The model under review builds one solid part; all positions refer to its coordinate system, in mm. Face numbers are marked on the shaded views. A direction names the side the tool comes from. Give positions to 0.01 mm unless a question says otherwise; leave off trailing zeros. Loops run counter-clockwise (first coordinate to the right, second up) from the corner with the lowest first, then second, coordinate; pieces in that order, holes last. Notation, with made-up numbers: M 10.5,-2 L 33.5,-2 A17 ccw 33.5,22 Z; hole C 46,64 d6. An arc over 180 degrees is marked long. Return JSON: item names as keys, results as strings. Group by question number.
```python
from build123d import *

# Parameters (mm, degrees)
F0_W     = 127
F0_H     = 127
F1_DEPTH = 6.35
F4_DEPTH = 762


with BuildPart() as f1:
    # F0 (on Front) → F1 (new body)
    with BuildSketch(Plane.XZ):
        with Locations((5.181599, -1.836989)):
            Rectangle(F0_W, F0_H)
    extrude(amount=F1_DEPTH)

    # F3 (on face) → F4 (join)
    with BuildSketch(Plane(origin=(0, 0, 0), x_dir=(-1, 0, 0), z_dir=(0, 1, 0))):
        Polygon((-11.394211, -37.070461), (1.031012, -37.070461), (12.706903, -32.820784), (22.225176, -24.834005), (28.437787, -14.073446), (30.595405, -1.836989), (28.437787, 10.399467), (22.225176, 21.160026), (12.706903, 29.146805), (1.031012, 33.396482), (-11.394211, 33.396482), (-23.070102, 29.146805), (-32.588375, 21.160026), (-38.800986, 10.399467), (-40.958604, -1.836989), (-38.800986, -14.073446), (-32.588375, -24.834005), (-23.070102, -32.820784), align=None)
    extrude(amount=F4_DEPTH)


solid = f1.part
```
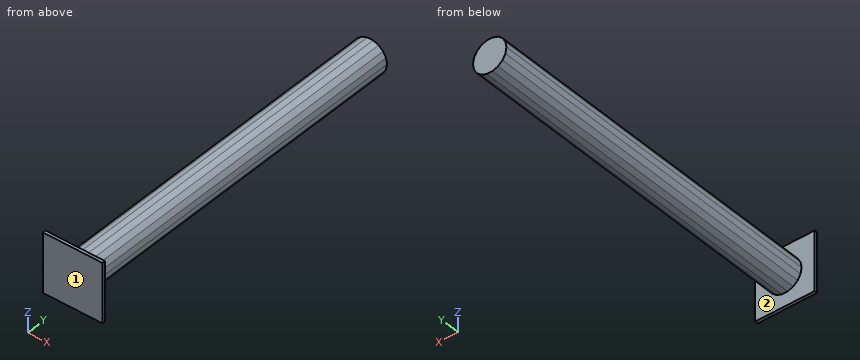
(1) Add section C-C (z = 50). Write out the cut boundary in (x, y).
(2) Add section A-A (y = 316.5). Write out the cut boundary in (x, z).
(3) Add section B-B (x = 53.5). Write out the cut boundary in (y, z), and give its area (3 significant figures).
(4) For probe 1 along Y at (x, z) = (29, -49); probe 2 along X at (y, z) = (649, 1); probe 3 along X at (y, z) = (596, -19), list the stretches that pass through material, from the lowest coordinate up.
(5) For the marked faces 1 and 2, list the 3-axis set-ups (+Z, -Z, +X, -X, +Y, -Y) from which the entire face can be reached by the end or side of a thin tool; tool diameter is ignored.
(6) For pin 1 (3 mm diameter, centred on x = 8, y = 550, fed in from +Z); pin 2 (3 mm diameter, centred on x = 25.5, z = -33.5, fed in from +Y); pin 3 (1.5 mm diameter, centred on x = 28, y = 161.5, fed in from +Z), all flat-tipped, find the tip position at first contact; note any pin that passes through.
Verdict:
{
 "1": {"outline": "M -58.32,-6.35 L 68.68,-6.35 L 68.68,0 L -58.32,0 Z"},
 "2": {"outline": "M -30.6,-1.84 L -28.44,-14.07 L -22.23,-24.83 L -12.71,-32.82 L -1.03,-37.07 L 11.39,-37.07 L 23.07,-32.82 L 32.59,-24.83 L 38.8,-14.07 L 40.96,-1.84 L 38.8,10.4 L 32.59,21.16 L 23.07,29.15 L 11.39,33.4 L -1.03,33.4 L -12.71,29.15 L -22.23,21.16 L -28.44,10.4 Z"},
 "3": {"outline": "M -6.35,-65.34 L 0,-65.34 L 0,61.66 L -6.35,61.66 Z", "area": "806 mm²"},
 "4": {"probe 1": "y = -6.35 to 0", "probe 2": "x = -30.1 to 40.46", "probe 3": "x = -25.59 to 35.96"},
 "5": {"face 1": "+Z, -Z, +X, -X, -Y", "face 2": "+Y"},
 "6": {"pin 1": "stops at z = 33.4", "pin 2": "stops at y = 0", "pin 3": "stops at z = 25.64"}
}
